CAD build for the part. Positions are in the model's coordinates, mm. Face numbers are marked on the shaded views. A direction names the side the tool comes from. Coordinates: 2 decimals unless noted, no trailing zeros. Loops run counter-clockwise (first coordinate to the right, second up) from the corner with the lowest first, then second, coordinate; pieces in that order, holes last. Notation, with made-up numbers: (29.25, 69.25) -> (40.25, 69.25) arc R5 cw to (40.25, 74.25) -> close; hole circle Ø7 at (-8.5, -36). An arc over 180 degrees is marked (long way). Return JSON: item names as keys, results as strings. Group by question number.
(1) Saw through at A-A on z = 6.5. Write the cut outline in (x, y).
(2) Saw through at B-B on x = 2.75. Write the cut outline in (y, z), then the cut area to 3 significant figures.
(3) Tool access for the marked faces 1 and 2: list every direction of +Z, -Z, +X, -X, +Y, -Y with a clear straight run to the whole face (end or side of a thin tool).
(4) Flat gauge pins, fed straight in: pin 1 Ø2 at (x, z) = (3, 7.5) entering from +Y; pin 2 Ø3 at (x, z) = (3, 8) entering from +Y; pin 3 Ø4 at (y, z) = (3, 3.5) entering from +X. Where does each tip first touch, or does it go through?
(5) Saw through at C-C on y = 3. Write the cut outline in (x, z), then the cut area to 3 significant figures.
(6) Probe L1, parallel to Z at x = -2, y = -2.5; L2, parallel to Y at x = 3.5, z = -1.5; L3, parallel to Y at x = -0.5, z = -1. List the from-to ranges inside material, lowest first.
```python
from build123d import *

# Parameters (mm, degrees)
BASE_SKETCH_R      = 4
BASE_EXTRUDE_DEPTH = 2
SKETCH2_R          = 2.4
TOP_EXTRUDE_DEPTH  = 10
TOP_FILLET_R       = 1.25


with BuildPart() as part:
    # Base Sketch → Base Extrude (new body)
    with BuildSketch(Plane.XY):
        Circle(BASE_SKETCH_R)
    extrude(amount=-BASE_EXTRUDE_DEPTH)

    # Sketch2 → Top Extrude (add)
    with BuildSketch(Plane.XY):
        Circle(SKETCH2_R)
    extrude(amount=TOP_EXTRUDE_DEPTH)

    # Top Fillet
    top_fillet_edges = [part.edges().sort_by_distance(p)[0] for p in [
        (-2.4, 0, 10),
    ]]
    fillet(top_fillet_edges, radius=TOP_FILLET_R)


solid = part.part
```
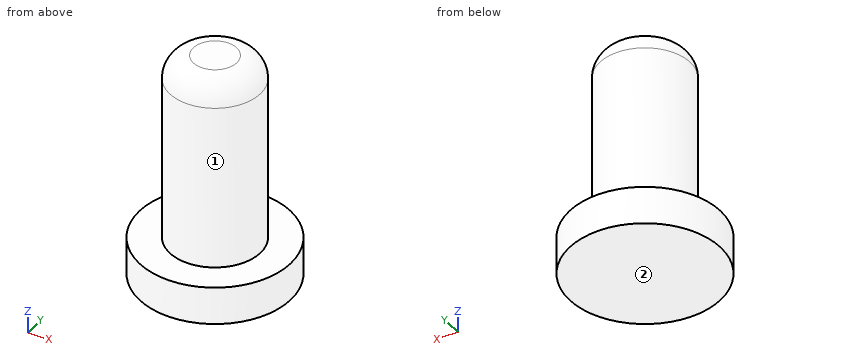
Geometry results:
{
 "1": {"outline": "circle Ø4.8 at (0, 0)"},
 "2": {"outline": "(-2.9, -2) -> (2.9, -2) -> (2.9, 0) -> (-2.9, 0) -> close", "area": "11.6 mm²"},
 "3": {"face 1": "+Z", "face 2": "-Z, +X, -X, +Y, -Y"},
 "4": {"pin 1": "y = 1.33", "pin 2": "y = 1.87", "pin 3": "x = 2.18"},
 "5": {"outline": "(-2.65, -2) -> (2.65, -2) -> (2.65, 0) -> (-2.65, 0) -> close", "area": "10.6 mm²"},
 "6": {"L1": "-2 to 0", "L2": "-1.94 to 1.94", "L3": "-3.97 to 3.97"}
}
